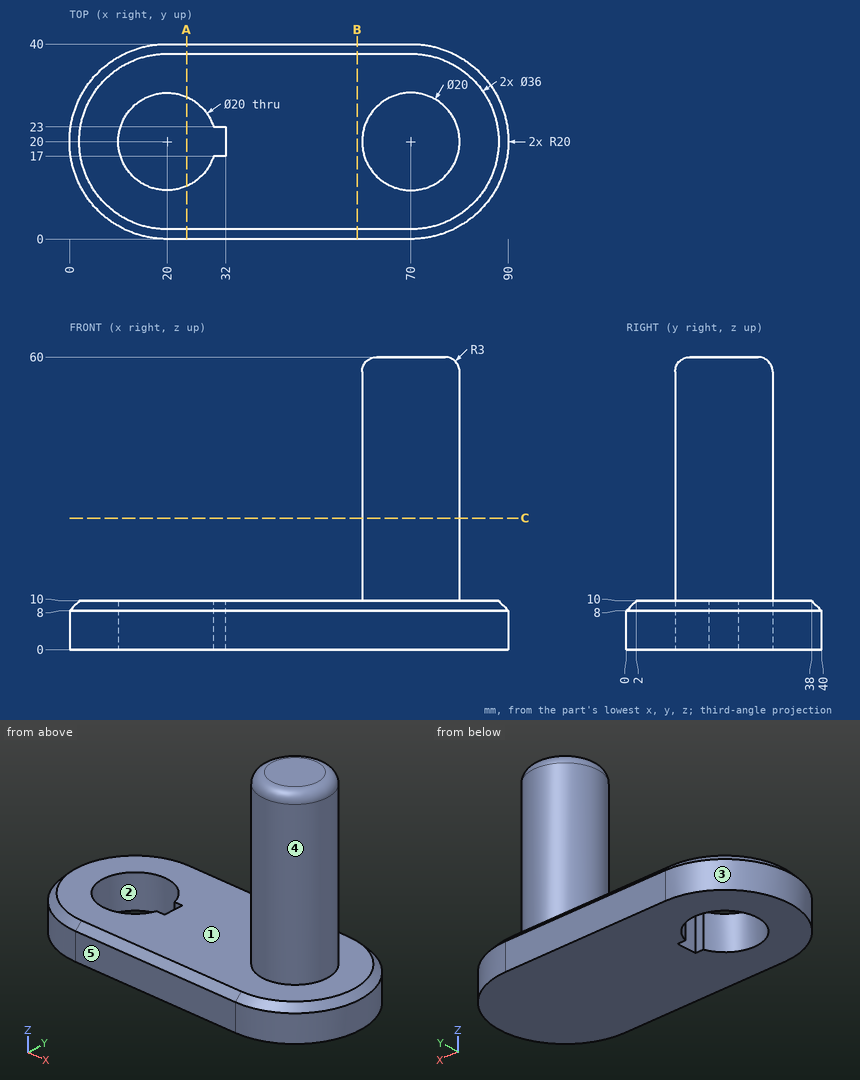
Part print with two shaded views. Sizes in mm from the minimum x, y, z corner. A direction names the side the tool comes from. Coordinates: 2 decimals unless noted, no trailing zeros. Write each loop counter-clockwise with the first axis right and the second up, starting at its lowest first coordinate (ties: lowest second). Pieces come first, ordered by that corner, then holes. Notation, with made-up numbers: (42, 26.25) - (68, 26.25) arc R19 ccw to (68, 51.25) - close; hole circle Ø7 at (-14.75, 60). An arc over 180 degrees is marked (long way). Use a Markdown table: item, result. Add a question column.
Item 1: Band-saw the part on A-A, the plane x = 24. Write the cut outline in (y, z), and give its area (3 significant figures).
Item 2: Two-plate mould, pull along X, no slides. Class the marked faces 1, 2 and 3: pulls with the +X half, pulls with the -X half, needs draft (parallel to the pull), parting line crosses it, or undercut.
Item 3: Drill centre lines: line 1 along Y through (x, z) = (20, 6.25); line 2 along X through (y, z) = (20, 5); line 3 along Z through (x, y) = (32, 26). Where is each one in solid material? Low to high.
Item 4: Drop flat-ended pins along their axis: pin 1 (3 mm diameter, centred on y = 21, z = 3.5, fed in from -X); pin 2 (5 mm diameter, centred on y = 9.5, z = 41, fed in from -X); pin 3 (6 mm diameter, centred on y = 10, z = 44.5, fed in from +X). Give the stop position or say it passes through.
Item 5: Band-saw the part on C-C, the plane z = 27. Write the cut outline in (x, y), and give its area (3 significant figures).
Item 6: Band-saw the part on B-B, the plane x = 59. Write the cut outline in (y, z).
Item 7: 3-axis set-ups, long thin cutter, end or side, ignore diameter. For the marked faces 4 and 5: which of +Z, -Z, +X, -X, +Y, -Y reach the whole face in a straight line?
A:
| question | item | result |
|---|---|---|
| 1 | outline | (0, 0) - (10.83, 0) - (10.83, 10) - (2, 10) - (0, 8) - close; (29.17, 0) - (40, 0) - (40, 8) - (38, 10) - (29.17, 10) - close |
| 1 | area | 213 mm² |
| 2 | face 1 | needs draft |
| 2 | face 2 | undercut |
| 2 | face 3 | pulls with the -X half |
| 3 | line 1 | y = 0 to 10, 30 to 40 |
| 3 | line 2 | x = 0 to 10, 32 to 90 |
| 3 | line 3 | z = 0 to 10 |
| 4 | pin 1 | stops at x = 0 |
| 4 | pin 2 | stops at x = 64 |
| 4 | pin 3 | stops at x = 77.14 |
| 5 | outline | circle Ø20 at (70, 20) |
| 5 | area | 314 mm² |
| 6 | outline | (0, 0) - (40, 0) - (40, 8) - (38, 10) - (2, 10) - (0, 8) - close |
| 7 | face 4 | +Z |
| 7 | face 5 | +Z, -Z, +X, -X, -Y |
